from build123d import *

# Parameters (mm, degrees)
SKETCH1_W                = 22.5
SKETCH1_H                = 7
BOSS_EXTRUDE1_DEPTH      = 1.5
SKETCH2_R                = 1.475
BOSS_EXTRUDE2_DEPTH      = 13.5
SKETCH3_R                = 1.05
BOSS_EXTRUDE3_DEPTH      = 10.5
SKETCH4_W                = 22.5
SKETCH4_H                = 2.5
SKETCH4_H_2              = 7
BOSS_EXTRUDE4_DEPTH      = 6
BOSS_EXTRUDE4_DEPTH_BACK = 1.5
SKETCH8_W                = 22.5
SKETCH8_H                = 9.5
BOSS_EXTRUDE7_DEPTH      = 2.61
SKETCH9_R                = 2.4
BOSS_EXTRUDE8_DEPTH      = 7.76
BOSS_EXTRUDE8_DEPTH_BACK = 1.5
SKETCH15_W               = 9.5
SKETCH15_H               = 3
BOSS_EXTRUDE11_DEPTH     = 4.5
SKETCH16_W               = 1.5
SKETCH16_H               = 9.5
CUT_EXTRUDE3_DEPTH       = 1.5


with BuildPart() as part:
    # Sketch1 → Boss-Extrude1 (new body)
    with BuildSketch(Plane(origin=(0, 0, 0), x_dir=(1, 0, 0), z_dir=(0, 1, 0))):
        with Locations((-28.93578967, -21.079480712)):
            Rectangle(SKETCH1_W, SKETCH1_H)
    extrude(amount=BOSS_EXTRUDE1_DEPTH)

    # Sketch2 → Boss-Extrude2 (add)
    with BuildSketch(Plane(origin=(0, 1.5, 0), x_dir=(1, 0, 0), z_dir=(0, 1, 0))):
        with Locations((-37.53578967, -19.579480712)):
            Circle(SKETCH2_R)
        with Locations((-20.33578967, -19.579480712)):
            Circle(SKETCH2_R)
    extrude(amount=BOSS_EXTRUDE2_DEPTH)

    # Sketch3 → Boss-Extrude3 (add)
    with BuildSketch(Plane(origin=(0, 1.5, 0), x_dir=(1, 0, 0), z_dir=(0, 1, 0))):
        with Locations((-37.88578967, -23.029480712)):
            Circle(SKETCH3_R)
        with Locations((-19.98578967, -23.029480712)):
            Circle(SKETCH3_R)
    extrude(amount=BOSS_EXTRUDE3_DEPTH)

    # Sketch4 → Boss-Extrude4 (add, two sides)
    with BuildSketch(Plane(origin=(0, 0, 0), x_dir=(-1, 0, 0), z_dir=(0, -1, 0))) as boss_extrude4_sk:
        with Locations((28.93578967, -25.829480712)):
            Rectangle(SKETCH4_W, SKETCH4_H)
        with Locations((28.93578967, -21.079480712)):
            Rectangle(SKETCH4_W, SKETCH4_H_2)
    extrude(amount=BOSS_EXTRUDE4_DEPTH)
    extrude(boss_extrude4_sk.sketch, amount=-BOSS_EXTRUDE4_DEPTH_BACK)

    # Sketch8 → Boss-Extrude7 (add)
    with BuildSketch(Plane(origin=(0, 1.5, 0), x_dir=(1, 0, 0), z_dir=(0, 1, 0))):
        with Locations((-28.93578967, -22.329480712)):
            Rectangle(SKETCH8_W, SKETCH8_H)
    extrude(amount=BOSS_EXTRUDE7_DEPTH)

    # Sketch9 → Boss-Extrude8 (add, two sides)
    with BuildSketch(Plane(origin=(0, -6, 0), x_dir=(-1, 0, 0), z_dir=(0, -1, 0))) as boss_extrude8_sk:
        with Locations((28.81078967, -25.489480712)):
            Circle(SKETCH9_R)
        with Locations((28.81078967, -17.519480712)):
            Circle(SKETCH9_R)
    extrude(amount=BOSS_EXTRUDE8_DEPTH)
    extrude(boss_extrude8_sk.sketch, amount=-BOSS_EXTRUDE8_DEPTH_BACK)

    # Sketch15 → Boss-Extrude11 (add)
    with BuildSketch(Plane.ZY.offset(40.18578967)):
        with Locations((22.329480712, -2.09)):
            Rectangle(SKETCH15_W, SKETCH15_H)
    extrude(amount=BOSS_EXTRUDE11_DEPTH)

    # Sketch16 → Cut-Extrude3 (cut)
    with BuildSketch(Plane(origin=(0, -0.59, 0), x_dir=(1, 0, 0), z_dir=(0, 1, 0))):
        with Locations((-42.43578967, -22.329480712)):
            Rectangle(SKETCH16_W, SKETCH16_H)
    extrude(amount=-CUT_EXTRUDE3_DEPTH, mode=Mode.SUBTRACT)


solid = part.part
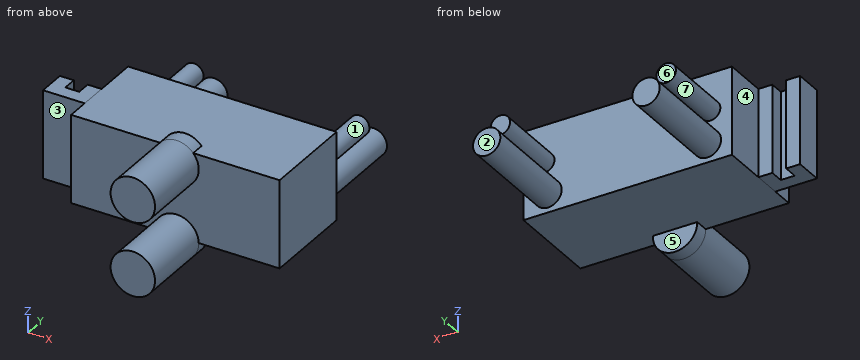
Part model, mm, in its own coordinate system. Face numbers are marked on the shaded views. A direction names the side the tool comes from. Round coordinates to 2 decimals unless told otherwise and drop trailing zeros. Write each loop counter-clockwise with the first axis right and the second up, starting at its lowest first coordinate (ties: lowest second). Pieces come first, ordered by that corner, then holes. Notation, with made-up numbers: M 47,43.5 L 70,43.5 A13 cw 70,57.5 Z; hole C 3,30.25 d11. An arc over 180 degrees is marked long. Return JSON: item names as keys, results as strings. Group by question number.
(1) Which spindle directions (+Z, -Z, +X, -X, +Y, -Y) get a long thin tool onto all of the face, cutting with end or side? Do the marked faces 3, 4, 5, 6 and 7. Say none if no direction does.
(2) Two-plate mould, pull along Z, no slides. Class the marked faces 1 and 2: +Z half, -Z half, draft (parallel to the pull), parting line (faces both ways), or undercut.
(3) Saw through at A-A on z = 21.5. Write the cut outline in (x, y), then the cut area to 3 significant figures.
(4) Saw through at D-D on y = -3. Write the cut outline in (x, z).
(5) Drill centre lines: probe 1 along Y at (x, z) = (-38.5, 26); probe 2 along X at (y, z) = (-2, 19); probe 3 along Y at (x, z) = (-29.5, 23.5). Where is each one in solid material? Low to high.
(6) Saw through at B-B on x = -30.25. Write the cut outline in (y, z).
(7) Saw through at C-C on y = 10.75. Write the cut outline in (x, z) (3 decimals).
(8) Pin check, flat tips, straight feed: pin 1 Ø3.5 at (x, y) = (-41.5, -1.5) entering from +Z; pin 2 Ø1.1 at (x, z) = (-19.5, 23) entering from +Y; pin 3 Ø1.2 at (y, z) = (-4.5, 20) entering from -X; pin 4 Ø6 at (y, z) = (4.5, 20.5) entering from +X. Stop position of each tip, or through.
Returned:
{
 "1": {"face 3": "+Z, -Z, -X, -Y", "face 4": "+Z, -Z, -X, +Y", "face 5": "-Z, +X, -X, +Y", "face 6": "+Z, +X, -X, +Y", "face 7": "+Y"},
 "2": {"face 1": "undercut", "face 2": "draft"},
 "3": {"outline": "M -44.69,-3.59 L -40.19,-3.59 L -40.19,-6 L -17.69,-6 L -17.69,4.11 L -40.19,4.11 L -40.19,-0.59 L -41.69,-0.59 L -41.69,-2.09 L -43.19,-2.09 L -43.19,-0.59 L -44.69,-0.59 Z", "area": "239 mm²"},
 "4": {"outline": "M -44.69,17.58 L -17.69,17.58 L -17.69,27.08 L -44.69,27.08 Z"},
 "5": {"probe 1": "-6 to 4.11", "probe 2": "-44.69 to -43.19, -41.69 to -17.69", "probe 3": "-13.76 to 4.11"},
 "6": {"outline": "M -13.76,15.6 L -4.5,15.6 L -4.5,17.58 L 4.11,17.58 L 4.11,27.08 L -4.5,27.08 L -4.5,27.41 L -13.76,27.41 L -13.76,23.57 L -6,23.57 L -6,19.44 L -13.76,19.44 Z"},
 "7": {"outline": "C -37.536,19.579 d2.95; C -37.886,23.029 d2.1; C -20.336,19.579 d2.95; C -19.986,23.029 d2.1"},
 "8": {"pin 1": "z = 27.08", "pin 2": "y = 12", "pin 3": "x = -40.19", "pin 4": "x = -17.69"}
}
